```python
from build123d import *

# Parameters (mm, degrees)
SKETCH_1_W          = 8
SKETCH_1_H          = 4.2
EXTRUDE_1_DEPTH     = 25
SKETCH_2_R          = 1.6
CUT_EXTRUDE_1_DEPTH = 57.789083458
SKETCH_3_R          = 1.6
CUT_EXTRUDE_2_DEPTH = 57.789083458
FILLET_7_R          = 1.5
CHAMFER_1_SIZE      = 5
FILLET_8_R          = 10
SKETCH1_W           = 19
SKETCH1_H           = 8.5
CUT_EXTRUDE1_DEPTH  = 7
CHAMFER1_START      = -19
CHAMFER1_OUTLINE_W  = 27
CHAMFER1_OUTLINE_H  = 17
CHAMFER1_DEPTH      = 4.338795771
CUT_EXTRUDE3_DEPTH  = 57.789083458
FILLET7_R           = 30
FILLET8_R           = 10


with BuildPart() as part:
    # Эскиз1 → Бобышка-Вытянуть1 (new body)
    with BuildSketch(Plane(origin=(0, 0, 0), x_dir=(1, 0, 0), z_dir=(0, 1, 0))):
        Polygon((-10, -30), (0, -30), (0, -50), (10, -50), (10, 50), (0, 50), (0, 30), (-10, 30), align=None)
        with Locations((4, 25)):
            Rectangle(SKETCH_1_W, SKETCH_1_H, mode=Mode.SUBTRACT)
        with Locations((4, -8)):
            Rectangle(SKETCH_1_W, SKETCH_1_H, mode=Mode.SUBTRACT)
    extrude(amount=EXTRUDE_1_DEPTH)

    # Эскиз2 → Вырез-Вытянуть1 (cut, through all)
    with BuildSketch(Plane.ZY):
        with Locations((-45, 6.5)):
            Circle(SKETCH_2_R)
        with Locations((-45, 18.5)):
            Circle(SKETCH_2_R)
    extrude(amount=-CUT_EXTRUDE_1_DEPTH, mode=Mode.SUBTRACT)

    # Эскиз3 → Вырез-Вытянуть2 (cut, through all)
    with BuildSketch(Plane.ZY):
        with Locations((45, 6.5)):
            Circle(SKETCH_3_R)
        with Locations((45, 18.5)):
            Circle(SKETCH_3_R)
    extrude(amount=-CUT_EXTRUDE_2_DEPTH, mode=Mode.SUBTRACT)

    # Скругление7
    fillet_7_edges = [part.edges().sort_by_distance(p)[0] for p in [
        (0, 12.5, 5.9),
        (0, 12.5, 10.1),
        (8, 12.5, 10.1),
        (8, 12.5, 5.9),
        (0, 12.5, -22.9),
        (8, 12.5, -22.9),
        (8, 12.5, -27.1),
        (0, 12.5, -27.1),
    ]]
    fillet(fillet_7_edges, radius=FILLET_7_R)

    # Фаска1
    chamfer_1_edges = [part.edges().sort_by_distance(p)[0] for p in [
        (5, 25, 50),
        (5, 25, -50),
    ]]
    chamfer(chamfer_1_edges, length=CHAMFER_1_SIZE)

    # Скругление8
    fillet_8_edges = [part.edges().sort_by_distance(p)[0] for p in [
        (0, 12.5, 30),
        (0, 12.5, -30),
    ]]
    fillet(fillet_8_edges, radius=FILLET_8_R - 0.0001)  # a hair under: the kernel refuses the full size

    # Sketch1 → Cut-Extrude1 (cut)
    with BuildSketch(Plane.XZ):
        with Locations((-0.5, 8)):
            Rectangle(SKETCH1_W, SKETCH1_H)
        with Locations((-0.5, -25)):
            Rectangle(SKETCH1_W, SKETCH1_H)
    extrude(amount=-CUT_EXTRUDE1_DEPTH, mode=Mode.SUBTRACT)

    # Chamfer1: read off the stored shape, not the designer's step
    # Chamfer1 outline → Chamfer1 (cut)
    with BuildSketch(Plane(origin=(0, 0, 0), x_dir=(0, 1, 0), z_dir=(0.9555233585367056, 0, -0.29491543074368715)).offset(CHAMFER1_START)):
        with Locations((12.5, 20.5)):
            Rectangle(CHAMFER1_OUTLINE_W, CHAMFER1_OUTLINE_H)
    extrude(amount=CHAMFER1_DEPTH, mode=Mode.SUBTRACT)

    # Sketch3 → Cut-Extrude3 (cut, through all)
    with BuildSketch(Plane(origin=(0, 25, 0), x_dir=(1, 0, 0), z_dir=(0, 1, 0))):
        with BuildLine():
            Line((0, 35), (0, 45))
            Line((0, 45), (-16.541380551, 45))
            Line((-16.541380551, 45), (-16.541380551, -45))
            Line((-16.541380551, -45), (0, -45))
            ThreePointArc((0, -45), (-2.523269625, -18.845948598), (-10, 6.343330813))
            ThreePointArc((-10, 6.343330813), (-7.428201086, 21.519007807), (0, 35))
        make_face()
    extrude(amount=-CUT_EXTRUDE3_DEPTH, mode=Mode.SUBTRACT)

    # Fillet7
    fillet7_edges = [part.edges().sort_by_distance(p)[0] for p in [
        (-10, 12.5, -6.343330813),
    ]]
    fillet(fillet7_edges, radius=FILLET7_R)

    # Fillet8
    fillet8_edges = [part.edges().sort_by_distance(p)[0] for p in [
        (0, 12.5, -35),
    ]]
    fillet(fillet8_edges, radius=FILLET8_R)


solid = part.part
```
Geometry check sheet. Reference: the model listing, model coordinates, mm. A direction names the side the tool comes from. Round coordinates to 2 decimals unless told otherwise and drop trailing zeros. Loops run counter-clockwise (first coordinate to the right, second up) from the corner with the lowest first, then second, coordinate; pieces in that order, holes last. Notation, with made-up numbers: M 51.25,80.5 L 63.25,80.5 A20 ccw 63.25,93.5 Z; hole C -5.5,68.25 d11. An arc over 180 degrees is marked long. Return JSON: item names as keys, results as strings. Group by question number.
(1) Set-up check for faces 5 (the face through (1, 3, 3.75)), 6 (the face through (5, 10, 50)), 7 (the face through (4, 16, 10.1)), 8 (the face through (0, 12, 45)), 9 (the face through (2, 0, -1)): record each of +Z, -Z, +X, -X, +Y, -Y from which the full face is reachable in a straight line by a thin tool's end or side.
(2) Go/stop test with flat-tipped pins: pin 1 (5 mm diameter, centred on x = 6.5, y = 22, fed in from -Z); pin 2 (7 mm diameter, centred on x = 3.5, z = 7.5, fed in from -Y); pin 3 (1 mm diameter, centred on y = 5, z = -4, fed in from -X); pin 4 (5.5 mm diameter, centred on y = 5, z = -25.5, fed in from -X). Record where each tip stops, or that it passes through.
(3) Scan lines: line 1 along Y through (x, z) = (6, -45); line 2 along Z through (x, y) = (5.75, 9.75); line 3 along Z through (x, y) = (2, 18.5). Record each from-to range of solid material in increasing order. Write a range as [from, to].
(4) Mould release check, pull along X, two halves, no side actions. Record for faces 1 (the face through (4, 16, -27.1)), 2 (the face through (4, 16, 5.9)), 3 (the face through (-2.523, 12.675, 18.85)), 4 (the face through (5, 23, 47)): pulls with the +X half, pulls with the -X half, needs draft (parallel to the pull), parting line crosses it, or undercut.
(5) Section check D-D, the plane z = -35. Enter the section's corners in (x, y).
(6) Section check B-B, the plane y = 9. Give the number of separate pieces and of enclosed holes in the cut face, and give its area (3 significant figures).
(7) Section check A-A, the plane x = 3. Enter the section's corners in (y, z), and give its area (3 significant figures).
Data:
{
 "1": {"face 5": "-X, -Y", "face 6": "+Z, +X, -X, +Y, -Y", "face 7": "+Y, -Y", "face 8": "+Z, -X, +Y, -Y", "face 9": "+Z, -Z, +X, -X, -Y"},
 "2": {"pin 1": "z = -50", "pin 2": "y = 7", "pin 3": "x = -8.89", "pin 4": "x = -6.64"},
 "3": {"line 1": "[0, 4.9], [8.1, 16.9], [20.1, 25]", "line 2": "[-50, -27.1], [-22.9, 5.9], [10.1, 50]", "line 3": "[-50, -46.6], [-43.4, -27.1], [-22.9, 5.9], [10.1, 43.4], [46.6, 50]"},
 "4": {"face 1": "undercut", "face 2": "undercut", "face 3": "pulls with the -X half", "face 4": "needs draft"},
 "5": {"outline": "M -0.56,0 L 10,0 L 10,25 L -0.56,25 Z"},
 "6": {"separate pieces": "1", "enclosed holes": "2", "area": "1,300 mm²"},
 "7": {"outline": "M 0,-50 L 20,-50 L 25,-45 L 25,-27.1 L 7,-27.1 L 7,-29.25 L 0,-29.25 Z; M 0,-20.75 L 7,-20.75 L 7,-22.9 L 25,-22.9 L 25,5.9 L 7,5.9 L 7,3.75 L 0,3.75 Z; M 0,12.25 L 7,12.25 L 7,10.1 L 25,10.1 L 25,45 L 20,50 L 0,50 Z; hole C 6.5,-45 d3.2; hole C 6.5,45 d3.2; hole C 18.5,-45 d3.2; hole C 18.5,45 d3.2", "area": "2,170 mm²"}
}
